Part print with two shaded views. Sizes in mm from the minimum x, y, z corner. Round coordinates to 2 decimals unless told otherwise and drop trailing zeros. Write each loop counter-clockwise with the first axis right and the second up, starting at its lowest first coordinate (ties: lowest second). Pieces come first, ordered by that corner, then holes.
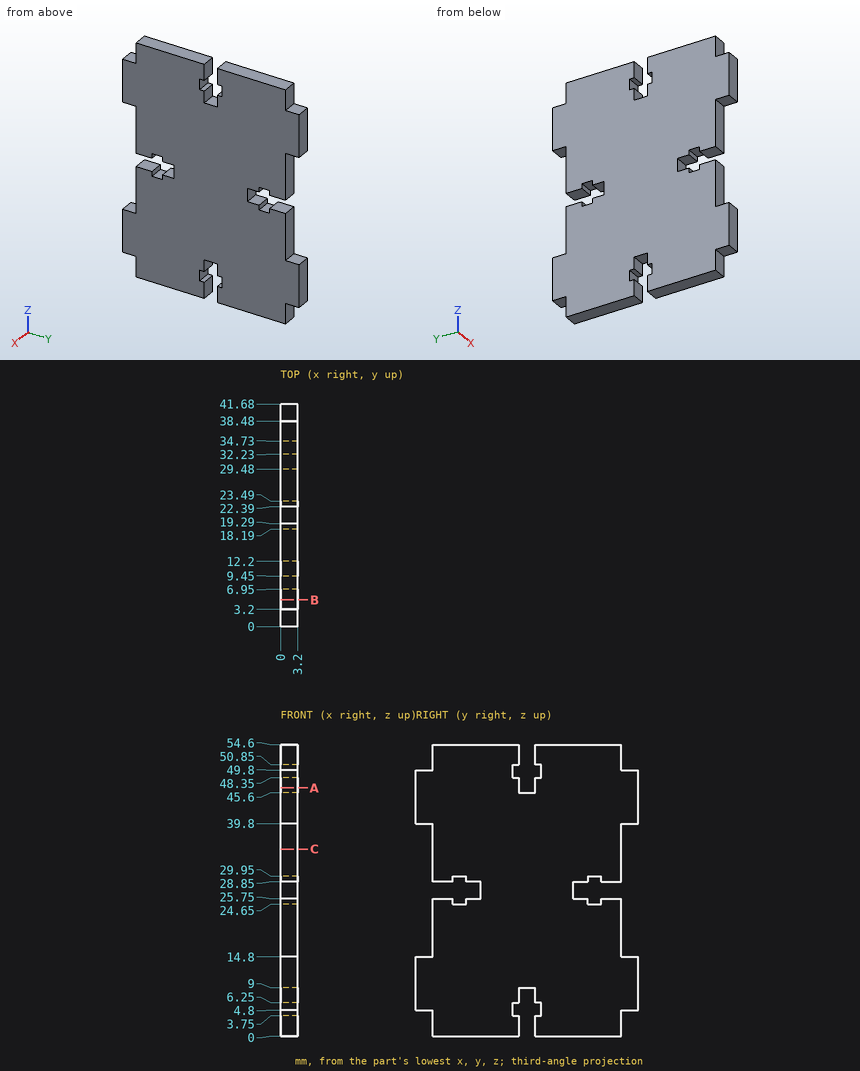
Q1. Cut at C-C on z = 35. Write the cut outline in (x, y), plus the area to 3 significant figures.
Values follow:
outline: (0, 3.2) - (3.2, 3.2) - (3.2, 38.48) - (0, 38.48) - close
area: 113 mm2
Q2. Cut at A-A on z = 46.5. Write the cut outline in (x, y).
Values follow:
outline: (0, 0) - (3.2, 0) - (3.2, 19.29) - (0, 19.29) - close; (0, 22.39) - (3.2, 22.39) - (3.2, 41.68) - (0, 41.68) - close
Q3. Wall check: L1, parallel to Z at x = 2.75, y = 30.5; L2, parallel to Y at x = 3.05, z = 48; L3, parallel to Z at x = 1.5, y = 9. Give the ranges that are in metal, low to high.
Values follow:
L1: z = 0 to 25.75, 28.85 to 54.6
L2: y = 0 to 19.29, 22.39 to 41.68
L3: z = 0 to 24.65, 29.95 to 54.6
Q4. Cut at B-B on y = 5. Write the cut outline in (x, z).
Values follow:
outline: (0, 0) - (3.2, 0) - (3.2, 25.75) - (0, 25.75) - close; (0, 28.85) - (3.2, 28.85) - (3.2, 54.6) - (0, 54.6) - close
Q5. Drop flat-ended pins along their axis: pin 1 (1.2 mm diameter, centred on x = 2, y = 23, fed in from -Z); pin 2 (0.5 mm diameter, centred on x = 1.5, z = 29.5, fed in from -Y); pin 3 (1.6 mm diameter, centred on x = 2, z = 52.5, fed in from +Y); pin 4 (1 mm diameter, centred on x = 2, y = 2.5, fed in from -Z). Give the stop position or say it passes through.
Values follow:
pin 1: stops at z = 0
pin 2: stops at y = 3.2
pin 3: stops at y = 38.48
pin 4: stops at z = 4.8
